CAD build for the part. Positions are in the model's coordinates, mm. Face numbers are marked on the shaded views. Give positions to 0.01 mm unless a question says otherwise; leave off trailing zeros. Order: outer loops, then holes, each group sorted by start corner. A loop starts at its lowest first (then second) coordinate and runs counter-clockwise, first axis right, second up.
Item 1: Two-plate mould, pull along X, no slides. Class the marked faces 1, 2 and 3: released by +X, released by -X, zero draft, split by the parting line, or undercut.
Item 2: Wall check: L1, parallel to Z at x = -3, y = 1.25; L2, parallel to X at y = 1.25, z = 2.75; L3, parallel to Y at x = 0, z = 6. Give the ranges that are in metal, low to high.
Item 3: Band-saw the part on A-A on z = 10. Give the cut face in (x, y), plus the area to 3 significant figures.
Item 4: Flat gauge pins, fed straight in: P1, Ø2, axis at x = 0, y = -1.5, coming from the +Z side; P2, Ø2, axis at y = -0.5, z = 14.5, coming from the -X side; P3, Ø2, axis at x = -3, z = 14.5, coming from the +Y side. Where does each tip first touch, or does it go through?
Item 5: Band-saw the part on B-B on z = 5.25. Give the cut face in (x, y), plus the area to 3 significant figures.
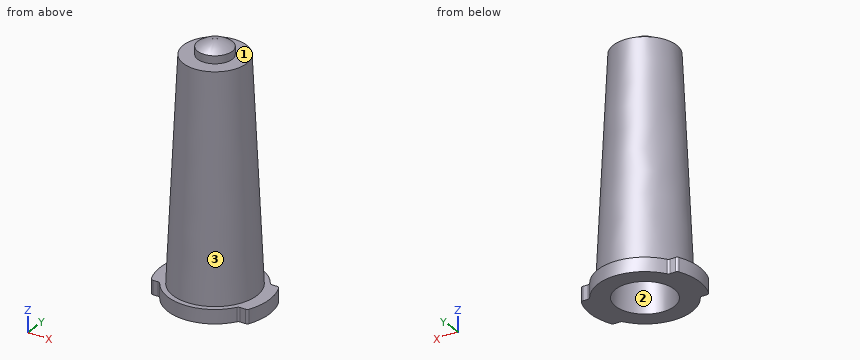
Autodesk Inventor part; units mm, degrees
ref_plane "YZ Plane" through (0, 0, 0) normal (1, 0, 0) x (0, 1, 0)
ref_plane "XZ Plane" through (0, 0, 0) normal (0, 1, 0) x (-1, 0, 0)
ref_plane "XY Plane" through (0, 0, 0) normal (0, 0, 1) x (1, 0, 0)
sketch "Sketch1" plane through (0, 0, 0) normal (0, 0, 1) x (1, 0, 0)
  circle A0 centre (0, 0) radius 3.365
  dimension "d0" = 6.73
sketch "Sketch2" plane through (0, 0, 0) normal (0, 1, 0) x (-1, 0, 0)
  line L0 (0, -3.16) -> (0, 18.96)
  line L1 (0, 0) -> (-2.26, 0)
  line L2 (0, 0) -> (-3, 0)
  line L3 (-3, 0) -> (-2.26, 15.8)
  line L4 (-2.26, 15.8) -> (0, 15.8)
  line L5 (0, 0) -> (0, 15.8)
  dimension "d3" = 2.26
  dimension "d5" = 2.26
  dimension "d6" = 3
  dimension "d7" = 15.8
revolve "Revolution1" add sketch "Sketch2" angle 360 about axis through (0, 0, -10) along (0, 0, 1)
sketch "Sketch3" plane through (0, 0, 0) normal (0, 0, -1) x (-1, 0, 0)
  circle A0 centre (0, 0) radius 3
extrude "Extrusion1" add sketch "Sketch1" against normal blind 1
sketch "Sketch4" plane through (0, 0, 0) normal (0, 0, 1) x (1, 0, 0)
  circle A0 centre (0, 0) radius 3.915
  line L0 (0, 1.75) -> (3.5021, 1.75)
  line L1 (8.4729, 1.75) -> (8.4729, -1.75)
  line L2 (3.5021, -1.75) -> (0, -1.75)
  line L3 (0, -1.75) -> (0, 1.75)
  point P0 (0, 0)
  dimension "d11" = 7.83
  dimension "d12" = 3.5
extrude "Extrusion2" add sketch "Sketch4" against normal blind 1 contours A0 L2 L3 L0 picked at (1.305, 0)
fillet "Fillet1" radius 0.2 4 edges at (2.8741, 1.75, -0.5) (2.8741, -1.75, -0.5) (3.5021, 1.75, -0.5) (3.5021, -1.75, -0.5)
mirror "Mirror1" about plane through (0, 0, 0) normal (1, 0, 0) of "Extrusion2", "Fillet1"
sketch "Sketch5" plane through (0, 0, -1) normal (0, 0, -1) x (-1, 0, 0)
  arc A0 (-2.817, -1.8406) -> (2.817, -1.8406) centre (0, 0) ccw
  circle A1 centre (0, 0) radius 0.205
  dimension "d16" = 0.41
extrude "Extrusion3" [suppressed]
sketch "Sketch6" plane through (0, 0, 0) normal (1, 0, 0) x (0, 1, 0)
  line L0 (0, -10.88) -> (0, 58.28)
  line L1 (2.26, 15.8) -> (-2.26, 15.8)
  line L2 (0, 16.3531) -> (1.235, 16.3531)
  line L3 (1.235, 16.3531) -> (1.235, 15.8)
  line L4 (1.235, 15.8) -> (0, 15.8)
  line L5 (0, 15.8) -> (0, 16.3531)
  arc A0 (1.235, 16.3531) -> (0, 16.8) centre (0, 14.87) ccw
  line L6 (0, 16.8) -> (0, 16.3531)
  point P0 (0, 0)
  dimension "d19" = 1.235
revolve "Revolution2" add sketch "Sketch6" angle 360 about axis through (0, 0, -10) along (0, 0, 1)
sketch "Sketch9" plane through (0, 0, 0) normal (1, 0, 0) x (0, 1, 0)
  line L0 (0, -10.88) -> (0, 58.28)
  line L1 (2.26, 15.8) -> (-2.26, 15.8)
  line L2 (3, 0) -> (2.26, 15.8)
  line L3 (-1.6334, -1) -> (1.6334, -1)
  line L4 (0, 18.0112) -> (0, -1)
  line L5 (2.1, -1) -> (1.36, 14.8)
  line L6 (0.205, 18.0112) -> (0, 18.0112)
  line L7 (0, -1) -> (2.1, -1)
  line L8 (1.36, 14.8) -> (0.205, 14.8)
  line L9 (0.205, 14.8) -> (0.205, 18.0112)
  arc A0 (1.235, 16.3531) -> (-1.235, 16.3531) centre (0, 14.87) ccw
  line L10 (0.205, 16.7891) -> (1.36, 14.8)
  dimension "d37" = 2.1
  dimension "d38" = 1
  dimension "d40" = 0.205
revolve "Revolution3" cut sketch "Sketch9" angle 360 about axis through (0, 0, -10) along (0, 0, 1)
properties part number "Luer_Female"
The answers:
1. face 1: zero draft
1. face 2: undercut
1. face 3: split by the parting line
2. L1: z = -1 to 0
2. L2: x = -2.58 to -1.46, 1.46 to 2.58
2. L3: y = -2.72 to -1.77, 1.77 to 2.72
3. outline: circle Ø5.06 at (0, 0); hole circle Ø3.17 at (0, 0)
3. area: 12.2 mm2
4. P1: stops at z = 16.73
4. P2: stops at x = -2.36
4. P3: stops at y = 1.18
5. outline: circle Ø5.51 at (0, 0); hole circle Ø3.61 at (0, 0)
5. area: 13.6 mm2
